Build history of the part. All positions in model axes, mm. Round coordinates to 2 decimals unless told otherwise and drop trailing zeros. Write each loop counter-clockwise with the first axis right and the second up, starting at its lowest first coordinate (ties: lowest second). Pieces come first, ordered by that corner, then holes. Notation, with made-up numbers: (57.25, 83) -> (61.25, 83) arc R21 cw to (61.25, 119) -> close; hole circle Ø3 at (12, -21). An arc over 180 degrees is marked (long way). One line per question, with ' | ' between items.
from build123d import *

# Parameters (mm, degrees)
F1_DEPTH = 6


with BuildPart() as f1:
    # F0 (on Top) → F1 (new body)
    with BuildSketch(Plane.XY):
        with BuildLine():
            Line((95, 262.1821570396), (0, 262.1821570396))
            Line((0, 262.1821570396), (-95, 262.1821570396))
            ThreePointArc((-95, 262.1821570396), (-98.5355339059, 260.7176909456), (-100, 257.1821570396))
            Line((-100, 257.1821570396), (-100, 95.3790545464))
            add(Edge.make_bspline(
                [(-140.6018761806, -209.8051889464), (-145.28862702, -136.7092151999), (-151.7930566351, -23.6301706956), (-115.64488398, 25.6274545282), (-97.9540393108, 76.553678361), (-99.4446328149, 90.2689875565), (-100, 95.3790545464)],
                knots=[0.0173618711, 0.0173618711, 0.0173618711, 0.0173618711, 0.4243124, 0.6579372091, 0.8725538192, 1, 1, 1, 1], degree=3))
            ThreePointArc((-140.6018761806, -209.8051889464), (-137.4634707904, -216.4591114866), (-130.6223684602, -219.1653251648))
            Line((-130.6223684602, -219.1653251648), (130.6223684602, -219.1653251648))
            ThreePointArc((130.6223684602, -219.1653251648), (137.4634707904, -216.4591114866), (140.6018761806, -209.8051889464))
            add(Edge.make_bspline(
                [(140.6018761806, -209.8051889464), (145.28862702, -136.7092151999), (151.7930566351, -23.6301706956), (115.64488398, 25.6274545282), (97.9540393108, 76.553678361), (99.4446328149, 90.2689875565), (100, 95.3790545464)],
                knots=[0.0173618711, 0.0173618711, 0.0173618711, 0.0173618711, 0.4243124, 0.6579372091, 0.8725538192, 1, 1, 1, 1], degree=3))
            Line((100, 95.3790545464), (100, 175.0877600908))
            ThreePointArc((100, 175.0877600908), (101.4644660941, 178.6232939968), (105, 180.0877600908))
            Line((105, 180.0877600908), (135, 180.0877600908))
            ThreePointArc((135, 180.0877600908), (138.5355339059, 181.5522261849), (140, 185.0877600908))
            Line((140, 185.0877600908), (140, 217.1821570396))
            ThreePointArc((140, 217.1821570396), (138.5355339059, 220.7176909456), (135, 222.1821570396))
            Line((135, 222.1821570396), (105, 222.1821570396))
            ThreePointArc((105, 222.1821570396), (101.4644660941, 223.6466231337), (100, 227.1821570396))
            Line((100, 227.1821570396), (100, 257.1821570396))
            ThreePointArc((100, 257.1821570396), (98.5355339059, 260.7176909456), (95, 262.1821570396))
        make_face()
        Polygon((-113.0212247372, -77.5594741106), (-102.2047810256, -89.4264161587), (-102.2047810256, -114.4264161587), (-113.0212247372, -126.2933582067), (-123.8376684487, -114.4264161587), (-123.8376684487, -89.4264161587), align=None, mode=Mode.SUBTRACT)
        Polygon((-76.974330689, -177.1341983843), (-76.974330689, -152.1341983843), (-66.1578869775, -140.2672563362), (-55.3414432659, -152.1341983843), (-55.3414432659, -177.1341983843), (-66.1578869775, -189.0011404323), align=None, mode=Mode.SUBTRACT)
        Polygon((-34.964894978, -112.7157764564), (-34.964894978, -92.3640566064), (-30.1484465599, -87.0798323475), (-25.3319981418, -92.3640566064), (-25.3319981418, -112.7157764564), (-30.1484465599, -118.0000007153), align=None, mode=Mode.SUBTRACT)
        Polygon((-64.1132891178, -15.046416223), (-53.2968454063, -26.9133582711), (-53.2968454063, -51.9133582711), (-64.1132891178, -63.7803003192), (-74.9297328293, -51.9133582711), (-74.9297328293, -26.9133582711), align=None, mode=Mode.SUBTRACT)
        Polygon((-39.5913329997, 5.2842242589), (-39.5913329997, 25.6359441089), (-34.7748845816, 30.9201683677), (-29.9584361635, 25.6359441089), (-29.9584361635, 5.2842242589), (-34.7748845816, 0), align=None, mode=Mode.SUBTRACT)
        Polygon((-1.0179981434, -173.7170352519), (-1.0179981434, -148.7170352519), (9.7984455681, -136.8500932038), (20.6148892796, -148.7170352519), (20.6148892796, -173.7170352519), (9.7984455681, -185.5839772999), align=None, mode=Mode.SUBTRACT)
        Polygon((40.3145010493, -114.2058925758), (40.3145010493, -93.8541727258), (45.1309494674, -88.5699484669), (49.9473978855, -93.8541727258), (49.9473978855, -114.2058925758), (45.1309494674, -119.4901168346), align=None, mode=Mode.SUBTRACT)
        Polygon((78.761510551, -136.8500932038), (89.5779542625, -148.7170352519), (89.5779542625, -173.7170352519), (78.761510551, -185.5839772999), (67.9450668395, -173.7170352519), (67.9450668395, -148.7170352519), align=None, mode=Mode.SUBTRACT)
        Polygon((120.0424358249, -80.2271872759), (130.8588795364, -92.094129324), (130.8588795364, -117.094129324), (120.0424358249, -128.961071372), (109.2259921134, -117.094129324), (109.2259921134, -92.094129324), align=None, mode=Mode.SUBTRACT)
        Polygon((1.0265997163, -48.4961951387), (1.0265997163, -23.4961951387), (11.8430434278, -11.6292530907), (22.6594871393, -23.4961951387), (22.6594871393, -48.4961951387), (11.8430434278, -60.3631371868), align=None, mode=Mode.SUBTRACT)
        Polygon((30.1835480056, 5.2842242589), (30.1835480056, 25.6359441089), (34.9999964237, 30.9201683677), (39.8164448418, 25.6359441089), (39.8164448418, 5.2842242589), (34.9999964237, 0), align=None, mode=Mode.SUBTRACT)
        Polygon((78.761510551, -11.6292530907), (89.5779542625, -23.4961951387), (89.5779542625, -48.4961951387), (78.761510551, -60.3631371868), (67.9450668395, -48.4961951387), (67.9450668395, -23.4961951387), align=None, mode=Mode.SUBTRACT)
        Polygon((-74.0937069058, 64.5764083862), (-74.0937069058, 89.5764083862), (-63.2772631943, 101.4433504343), (-52.4608194828, 89.5764083862), (-52.4608194828, 64.5764083862), (-63.2772631943, 52.7094663382), align=None, mode=Mode.SUBTRACT)
        Polygon((-39.591331137, 130.4391115935), (-39.591331137, 150.7908314435), (-34.7748827189, 156.0750557024), (-29.9584343008, 150.7908314435), (-29.9584343008, 130.4391115935), (-34.7748827189, 125.1548873346), align=None, mode=Mode.SUBTRACT)
        Polygon((-63.2772631943, 229.4433504343), (-52.4608194828, 217.5764083862), (-52.4608194828, 192.5764083862), (-63.2772631943, 180.7094663382), (-74.0937069058, 192.5764083862), (-74.0937069058, 217.5764083862), align=None, mode=Mode.SUBTRACT)
        Polygon((-10.0937069058, 64.5764083862), (-10.0937069058, 89.5764083862), (0.7227368057, 101.4433504343), (11.5391805172, 89.5764083862), (11.5391805172, 64.5764083862), (0.7227368057, 52.7094663382), align=None, mode=Mode.SUBTRACT)
        Polygon((53.9062930942, 64.5764083862), (53.9062930942, 89.5764083862), (64.7227368057, 101.4433504343), (75.5391805172, 89.5764083862), (75.5391805172, 64.5764083862), (64.7227368057, 52.7094663382), align=None, mode=Mode.SUBTRACT)
        Polygon((30.1835480056, 130.4391115935), (30.1835480056, 150.7908314435), (34.9999964237, 156.0750557024), (39.8164448418, 150.7908314435), (39.8164448418, 130.4391115935), (34.9999964237, 125.1548873346), align=None, mode=Mode.SUBTRACT)
        Polygon((-10.0937069058, 192.5764083862), (-10.0937069058, 217.5764083862), (0.7227368057, 229.4433504343), (11.5391805172, 217.5764083862), (11.5391805172, 192.5764083862), (0.7227368057, 180.7094663382), align=None, mode=Mode.SUBTRACT)
        Polygon((53.9062930942, 192.5764083862), (53.9062930942, 217.5764083862), (64.7227368057, 229.4433504343), (75.5391805172, 217.5764083862), (75.5391805172, 192.5764083862), (64.7227368057, 180.7094663382), align=None, mode=Mode.SUBTRACT)
    extrude(amount=F1_DEPTH)


solid = f1.part
(1) Drop flat-ended pins along their axis: pin 1 (1.8 mm diameter, centred on y = 74, z = 1.5, fed in from -X); pin 2 (1.8 mm diameter, centred on y = 142.5, z = 3.5, fed in from -X); pin 3 (1.8 mm diameter, centred on y = 72, z = 2, fed in from +X). Give the stop position or say it passes through.
Calculated:
pin 1: x = -100.85 | pin 2: x = -100 | pin 3: x = 101.29
(2) Wall check: line 1 (X direction, y = -27, z = 2.5); line 2 (X direction, y = -39, z = 3.75); line 3 (Y direction, x = -7, z = 3.75). Give the ranges that are in metal, low to high. Write a range as from..to.
Calculated:
line 1: -140.7..-74.93, -53.3..1.03, 22.66..67.95, 89.58..140.7 | line 2: -142.71..-74.93, -53.3..1.03, 22.66..67.95, 89.58..142.71 | line 3: -219.17..61.18, 92.97..189.18, 220.97..262.18
(3) Slice it at A-A (y = 146). Write the cut outline in (x, z), then the cut area to 3 significant figures.
Calculated:
outline: (-100, 0) -> (-39.59, 0) -> (-39.59, 6) -> (-100, 6) -> close; (-29.96, 0) -> (30.18, 0) -> (30.18, 6) -> (-29.96, 6) -> close; (39.82, 0) -> (100, 0) -> (100, 6) -> (39.82, 6) -> close | area: 1,080 mm2
(4) Mould opens along X. For faces 1 (the flat face through (-2, -29, 0)), 2 (the flat face through (-118.354, -120.443, 2.958)) say: pulls with the +X half, pulls with the -X half, needs draft (parallel to the pull), parting line crosses it, or undercut.
Calculated:
face 1: needs draft | face 2: undercut
(5) Slice it at B-B (x = 114.5). State how many separate pieces and enclosed holes the cut face has, then the cut area to 3 significant figures.
Calculated:
separate pieces: 3 | enclosed holes: 0 | area: 1,550 mm2
